Source: three-view drawing plus pictorial views. Frame: mm from the lowest corner of the part. A direction names the side the tool comes from. Coordinates: 2 decimals unless noted, no trailing zeros. Write each loop counter-clockwise with the first axis right and the second up, starting at its lowest first coordinate (ties: lowest second). Pieces come first, ordered by that corner, then holes.
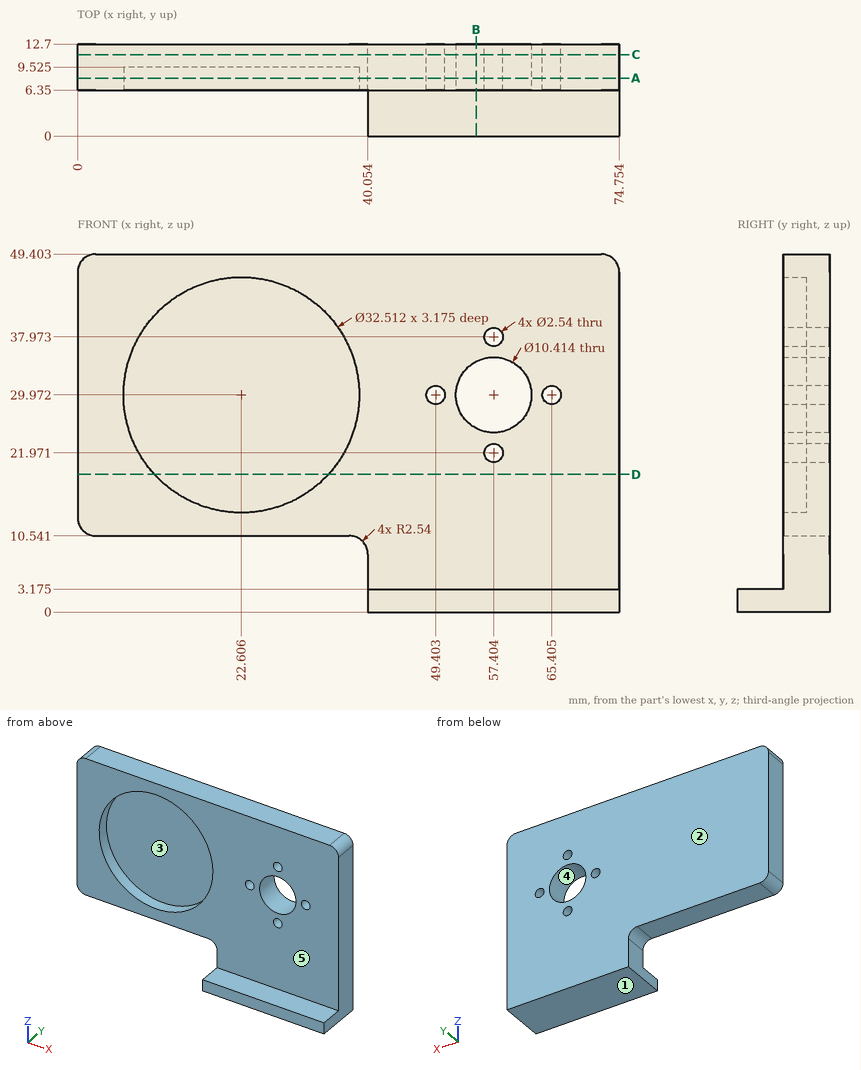
Item 1: Section query A-A, the plane y = 8. Return loops of the section in (x, z) (3 decimals).
Item 2: Section query B-B, the plane x = 55. Return loops of the section in (y, z) (3 decimals), then the cut area to 3 significant figures.
Item 3: Access query for the marked faces 4 and 5. Directions: +Z, -Z, +X, -X, +Y, -Y. A direction counts if a zero-diameter tool reaches every point of the face in a straight line with its end or side. Return the directions, or none.
Item 4: Material intervals for line 1 (Z direction, x = 72.5, y = 7.5); line 2 (Z direction, x = 42.5, y = 6.25) (3 decimals); line 3 (X direction, y = 10, z = 7), sorted ascending.
Item 5: Section query C-C, the plane y = 11.25. Return loops of the section in (x, z) (3 decimals).
Item 6: Pull-direction query (Z, two-part tool) for the marked faces 1, 2 and 3; classes: released by +Z, released by -Z, zero draft, split by the parting line, or undercut.
Item 7: Section query D-D, the plane z = 19. Return loops of the section in (x, y) (3 decimals), then the cut area to 3 significant figures.
Item 8: Pin query (flat end, axial travel): pin 1 Ø1.5 at (x, z) = (28, 23.5) entering from -Y (3 decimals); pin 2 Ø6 at (y, z) = (7.5, 44.5) entering from -X; pin 3 Ø5 at (x, y) = (28.5, 11) entering from -Z; pin 4 Ø5 at (x, y) = (64, 1.5) entering from +Z (3 decimals). Return the tip coordinate at first contact, or that it passes through.
The answers:
1. outline: (0, 13.081) arc R2.54 ccw to (2.54, 10.541) - (37.514, 10.541) arc R2.54 cw to (40.054, 8.001) - (40.054, 0) - (74.754, 0) - (74.754, 46.863) arc R2.54 ccw to (72.214, 49.403) - (2.54, 49.403) arc R2.54 ccw to (0, 46.863) - close; hole circle Ø32.512 at (22.606, 29.972); hole circle Ø2.54 at (49.403, 29.972); hole circle Ø10.414 at (57.404, 29.972); hole circle Ø2.54 at (57.404, 21.971); hole circle Ø2.54 at (57.404, 37.973); hole circle Ø2.54 at (65.405, 29.972)
2. outline: (0, 0) - (12.7, 0) - (12.7, 25.353) - (6.35, 25.353) - (6.35, 3.175) - (0, 3.175) - close; (6.35, 34.591) - (12.7, 34.591) - (12.7, 49.403) - (6.35, 49.403) - close
2. area: 275 mm2
3. face 4: +Y, -Y
3. face 5: +Z, +X, -X, -Y
4. line 1: z = 0 to 49.39
4. line 2: z = 0 to 3.175
4. line 3: x = 40.05 to 74.75
5. outline: (0, 13.081) arc R2.54 ccw to (2.54, 10.541) - (37.514, 10.541) arc R2.54 cw to (40.054, 8.001) - (40.054, 0) - (74.754, 0) - (74.754, 46.863) arc R2.54 ccw to (72.214, 49.403) - (2.54, 49.403) arc R2.54 ccw to (0, 46.863) - close; hole circle Ø2.54 at (49.403, 29.972); hole circle Ø10.414 at (57.404, 29.972); hole circle Ø2.54 at (57.404, 21.971); hole circle Ø2.54 at (57.404, 37.973); hole circle Ø2.54 at (65.405, 29.972)
6. face 1: released by -Z
6. face 2: zero draft
6. face 3: undercut
7. outline: (0, 6.35) - (10.611, 6.35) - (10.611, 9.525) - (34.601, 9.525) - (34.601, 6.35) - (74.754, 6.35) - (74.754, 12.7) - (0, 12.7) - close
7. area: 399 mm2
8. pin 1: stops at y = 9.525
8. pin 2: stops at x = 0
8. pin 3: stops at z = 10.54
8. pin 4: stops at z = 3.175
